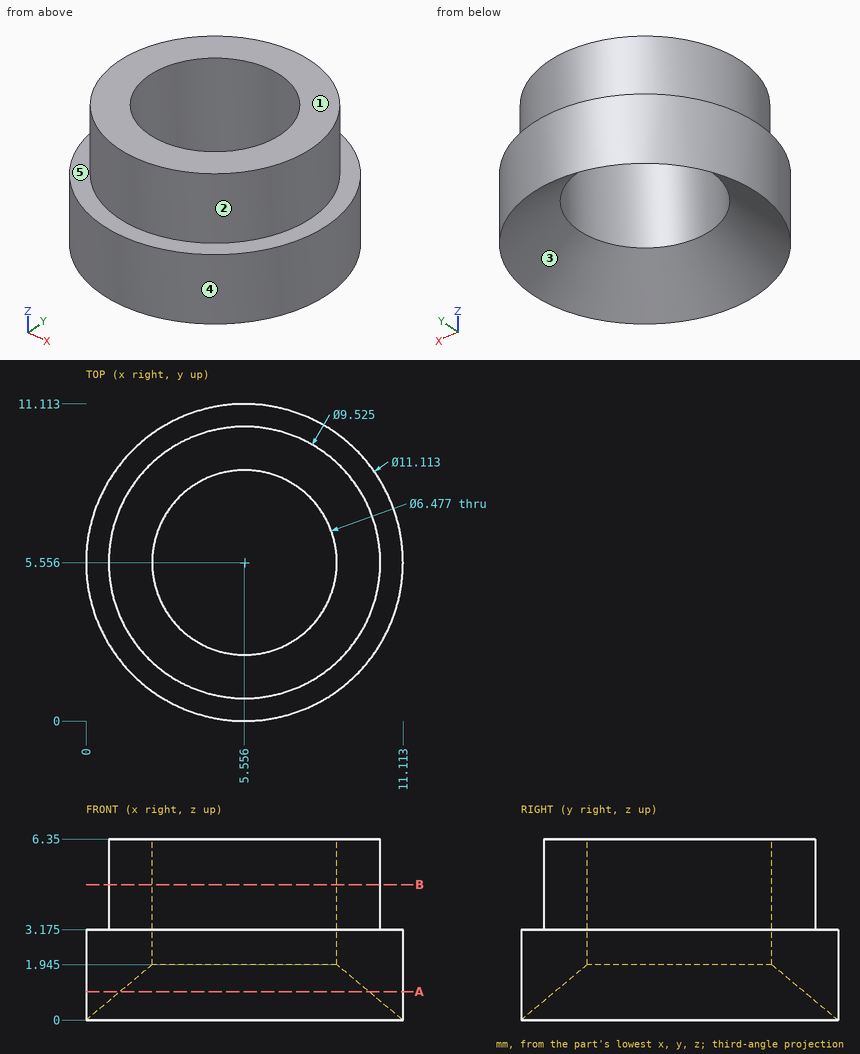
Check sheet for the drawn part. Datum: minimum x, y, z corner. Units: mm. A direction names the side the tool comes from. Give positions to 0.01 mm unless a question says otherwise; leave off trailing zeros. Order: outer loops, then holes, each group sorted by start corner. A loop starts at its lowest first (then second) coordinate and runs counter-clockwise, first axis right, second up. Notation, with made-up numbers: (-13, -20.75) -> (-6, -20.75) arc R22 ccw to (-6, -3.75) -> close; hole circle Ø3 at (23.5, 50). An arc over 180 degrees is marked (long way). Use a Markdown table: item, result.
1) Tool access check on the marked faces 1 and 2. Record the directions out of +Z, -Z, +X, -X, +Y, -Y that give a thin tool (end or side, any length) a straight path to the whole face; none if there is none.
Results:
| item | result |
|---|---|
| face 1 | +Z, +X, -X, +Y, -Y |
| face 2 | +Z |
2) Depth check by flat-ended pin: pin 1 Ø1 at (x, z) = (4.5, 1.5) entering from +Y (1 decimal); pin 2 Ø1 at (x, y) = (4.5, 3.5) entering from -Z. Enter the tip coordinate at first touch or a pass-through.
Results:
| item | result |
|---|---|
| pin 1 | y = 11.1 |
| pin 2 | through |
3) Material ranges on probe 1 along Y at (x, z) = (4.25, 4.5) (1 decimal); probe 2 along Y at (x, z) = (5.25, 3.25); probe 3 along X at (y, z) = (6.5, 5.5) (1 decimal), recorded low to high.
Results:
| item | result |
|---|---|
| probe 1 | 1 to 2.6, 8.5 to 10.1 |
| probe 2 | 0.8 to 2.33, 8.78 to 10.31 |
| probe 3 | 0.9 to 2.5, 8.7 to 10.2 |
4) Mould release check, pull along Y, two halves, no side actions. Record for the marked faces 3, 4 and 5: pulls with the +Y half, pulls with the -Y half, needs draft (parallel to the pull), parting line crosses it, or undercut.
Results:
| item | result |
|---|---|
| face 3 | undercut |
| face 4 | parting line crosses it |
| face 5 | needs draft |
5) Section check B-B, the plane z = 4.75. Record the boundary of the cut face in (x, y) (1 decimal).
Results:
| item | result |
|---|---|
| outline | circle Ø9.5 at (5.6, 5.6); hole circle Ø6.5 at (5.6, 5.6) |
6) Section check A-A, the plane z = 1. Record the boundary of the cut face in (x, y) (1 decimal).
Results:
| item | result |
|---|---|
| outline | circle Ø11.1 at (5.6, 5.6); hole circle Ø8.7 at (5.6, 5.6) |
